CAD build for the part. Positions are in the model's coordinates, mm. A direction names the side the tool comes from. Coordinates: 2 decimals unless noted, no trailing zeros. Loops run counter-clockwise (first coordinate to the right, second up) from the corner with the lowest first, then second, coordinate; pieces in that order, holes last. Notation, with made-up numbers: (-16.75, 82.5) -> (5.25, 82.5) arc R27 cw to (5.25, 119.5) -> close; hole circle Ø1 at (79, 81). An arc over 180 degrees is marked (long way). Write each question's results on one line, items separated by ' | '.
from build123d import *

# Parameters (mm, degrees)
SKETCH1_R           = 2.8702
BOSS_EXTRUDE1_DEPTH = 6.35
FILLET1_R           = 5.08


with BuildPart() as part:
    # Sketch1 → Boss-Extrude1 (new body)
    with BuildSketch(Plane.XY):
        Polygon((-133.35, 0), (-146.05, 0), (-146.05, -6.35), (-146.05, -9.05192086), (-179.812411975, -9.05192086), (-179.812411975, 2.216051439), (-195.472684717, 2.216051439), (-195.472684717, -16.678421964), (-195.472684717, -25.43652623), (-146.05, -25.43652623), (-133.35, -25.43652623), (-133.35, -6.35), align=None)
        with Locations((-186.939684717, -3.685756589)):
            Circle(SKETCH1_R, mode=Mode.SUBTRACT)
    extrude(amount=BOSS_EXTRUDE1_DEPTH)

    # Fillet1
    fillet1_edges = [part.edges().sort_by_distance(p)[0] for p in [
        (-133.35, -25.43652623, 3.175),
        (-195.472684717, -25.43652623, 3.175),
        (-195.472684717, 2.216051439, 3.175),
        (-179.812411975, 2.216051439, 3.175),
        (-179.812411975, -9.05192086, 3.175),
    ]]
    fillet(fillet1_edges, radius=FILLET1_R)


solid = part.part
1) Slice it at C-C (x = -141). Write the cut outline in (y, z), then the cut area to 3 significant figures.
Outcome:
outline: (-25.44, 0) -> (0, 0) -> (0, 6.35) -> (-25.44, 6.35) -> close | area: 162 mm^2
2) Slice it at B-B (z = 3.5). Write the cut outline in (x, y), then the cut area to 3 significant figures.
Outcome:
outline: (-195.47, -20.36) arc R5.08 ccw to (-190.39, -25.44) -> (-138.43, -25.44) arc R5.08 ccw to (-133.35, -20.36) -> (-133.35, 0) -> (-146.05, 0) -> (-146.05, -9.05) -> (-174.73, -9.05) arc R5.08 cw to (-179.81, -3.97) -> (-179.81, -2.86) arc R5.08 ccw to (-184.89, 2.22) -> (-190.39, 2.22) arc R5.08 ccw to (-195.47, -2.86) -> close; hole circle Ø5.74 at (-186.94, -3.69) | area: 1,270 mm^2
3) Pin check, flat tip, straight feed: pin 1 (3 mm diameter, centred on x = -161.5, z = 1, fed in from +Y). Stop position of the tip, or through.
Outcome:
pin 1: stops at y = -9.05
4) Two-plate mould, pull along X, no slides. Class faces 4 (the flat face through (-195.473, -11, 3)), 5 (the cylindrical face through (-178.285, -7.603, 3.219)), 6 (the flat face through (-165, -14, 6.35)), 7 (the flat face through (-146.05, -4, 3)): pulls with the +X half, pulls with the -X half, needs draft (parallel to the pull), parting line crosses it, or undercut.
Outcome:
face 4: pulls with the -X half | face 5: undercut | face 6: needs draft | face 7: undercut
5) Which spindle directions (+Z, -Z, +X, -X, +Y, -Y) get a long thin tool onto all of the face, cutting with end or side? Do faces 1 (the flat face through (-140, 0, 3)), 2 (the flat face through (-133.35, -10, 3)), 3 (the cylindrical face through (-181.26, 0.69, 3.22)). Say none if no direction does.
Outcome:
face 1: +Z, -Z, +X, +Y | face 2: +Z, -Z, +X, +Y, -Y | face 3: +Z, -Z, +Y
6) Slice it at D-D (y = -23.5). Write the cut outline in (x, z).
Outcome:
outline: (-194.38, 0) -> (-134.44, 0) -> (-134.44, 6.35) -> (-194.38, 6.35) -> close
7) Slice it at A-A (x = -188.5). Write the cut outline in (y, z), then the cut area to 3 significant figures.
Outcome:
outline: (-25.44, 0) -> (-6.09, 0) -> (-6.09, 6.35) -> (-25.44, 6.35) -> close; (-1.28, 0) -> (2.22, 0) -> (2.22, 6.35) -> (-1.28, 6.35) -> close | area: 145 mm^2
8) Drill centre lines: L1, parallel to X at y = -2.75, z = 0.5; L2, parallel to Y at x = -173, z = 1.75; L3, parallel to Y at x = -144, z = 5. Where is each one in solid material? Low to high. Write a range as from..to.
Outcome:
L1: x = -195.47..-189.65, -184.23..-179.81, -146.05..-133.35 | L2: y = -25.44..-9.05 | L3: y = -25.44..0
